Geometry check sheet. Reference: the model listing, model coordinates, mm. Coordinates: 2 decimals unless noted, no trailing zeros. Loops run counter-clockwise (first coordinate to the right, second up) from the corner with the lowest first, then second, coordinate; pieces in that order, holes last. Notation, with made-up numbers: (-4.75, -33.75) -> (31.25, -33.75) arc R33 cw to (31.25, -2.75) -> close; hole circle Ø3 at (49, -6). An arc over 180 degrees is marked (long way). Answer as a JSON object with one key per item and string values.
from build123d import *

# Parameters (mm, degrees)
F0_W     = 5.2
F0_H     = 226.71
F1_DEPTH = 2
F3_DEPTH = 4.5
F4_W     = 1.2
F4_H     = 2.1
F5_DEPTH = 25
F6_SIZE  = 1


with BuildPart() as f1:
    # F0 (on Top) → F1 (new body)
    with BuildSketch(Plane.XY):
        with Locations((2.6, 113.355)):
            Rectangle(F0_W, F0_H)
    extrude(amount=F1_DEPTH)

    # F2 (on face) → F3 (join)
    with BuildSketch(Plane.XY.offset(2)):
        Polygon((0, 226.71), (0, 0), (2, 0), (2, 224.71), (3.2, 224.71), (3.2, 0), (5.2, 0), (5.2, 226.71), align=None)
    extrude(amount=F3_DEPTH)

    # F4 (on face) → F5 (cut)
    with BuildSketch(Plane.XY.offset(2)):
        with Locations((2.6, 2.95)):
            Rectangle(F4_W, F4_H)
    extrude(amount=-F5_DEPTH, mode=Mode.SUBTRACT)

    # F6
    f6_edges = [f1.edges().sort_by_distance(p)[0] for p in [
        (2.6, 0, 2),
    ]]
    chamfer(f6_edges, length=F6_SIZE)


solid = f1.part
1. Section check A-A, the plane z = 3.25. Record the boundary of the cut face in (x, y), then the cut area to 3 significant figures.
Evaluation:
{"outline": "(0, 0) -> (2, 0) -> (2, 224.71) -> (3.2, 224.71) -> (3.2, 0) -> (5.2, 0) -> (5.2, 226.71) -> (0, 226.71) -> close", "area": "909 mm^2"}
2. Mould release check, pull along X, two halves, no side actions. Record for faces 1 (the face through (5.2, 112, 3)), 2 (the face through (2, 111, 4)), 3 (the face through (0, 115, 3)): released by +X, released by -X, zero draft, split by the parting line, or undercut.
Evaluation:
{"face 1": "released by +X", "face 2": "undercut", "face 3": "released by -X"}
3. Section check B-B, the plane y = 42.5. Record the boundary of the cut face in (x, z).
Evaluation:
{"outline": "(0, 0) -> (5.2, 0) -> (5.2, 6.5) -> (3.2, 6.5) -> (3.2, 2) -> (2, 2) -> (2, 6.5) -> (0, 6.5) -> close"}
4. Depth check by flat-ended pin: P1, Ø0.7, axis at x = 2.5, y = 1.5, coming from the +Z side. Enter the tip coordinate at first touch or a pass-through.
Evaluation:
{"P1": "stops at z = 2"}
5. Thickness scan on probe 1 along X at (y, z) = (214, 5.5); probe 2 along Y at (x, z) = (3, 1); probe 3 along Z at (x, y) = (2.75, 206). Record the ranges inside material, lowest first. Write a range as from..to.
Evaluation:
{"probe 1": "x = 0..2, 3.2..5.2", "probe 2": "y = 0..1.9, 4..226.71", "probe 3": "z = 0..2"}
